Could you check a few things on this model? Use its own coordinates, in mm. Give positions to 0.01 mm unless a question says otherwise; leave off trailing zeros. Order: outer loops, then holes, each group sorted by start corner. A loop starts at its lowest first (then second) coordinate and runs counter-clockwise, first axis right, second up. Notation, with made-up numbers: (-18.75, 23) -> (35.25, 23) arc R29 cw to (35.25, 46) -> close; hole circle Ø4 at (51.25, 69). An arc over 180 degrees is marked (long way). One line per item, written item: value.
```python
from build123d import *

# Parameters (mm, degrees)
CYLINDER_R     = 1.4
CYLINDER_DEPTH = 10
ARRAY001_COUNT = 3
SKETCH018_W    = 3.15
SKETCH018_H    = 2.3
SKETCH002_W    = 5
SKETCH002_H    = 6.8
ARRAY_Z_COUNT  = 6
ARRAY_Z_PITCH  = 1.6
SKETCH005_W    = 10
SKETCH005_H    = 2.2955317108


with BuildPart() as boltholes:
    # Cylinder → Cylinder (new body)
    with BuildSketch(Plane(origin=(0, 6, -1), x_dir=(1, 0, 0), z_dir=(0, 0, 1))):
        Circle(CYLINDER_R)
    extrude(amount=CYLINDER_DEPTH)

    # Array001: BoltHoles ×3 about axis
    array001_axis = Axis((0, 0, 0), (0, 0, 1))


with BuildPart() as boltholes_1:
    add(boltholes.part)
    for i in range(1, ARRAY001_COUNT):
        add(boltholes.part.rotate(array001_axis, i * 360 / ARRAY001_COUNT))


with BuildPart() as obj1:
    # Sketch018 → Revolution007 (revolve)
    with BuildSketch(Plane.XZ):
        with Locations((1.575, 5.7267413876)):
            Rectangle(SKETCH018_W, SKETCH018_H)
    revolve(axis=Axis((0, 0, 0), (0, 0, 1)))


with BuildPart() as obj2:
    # Sketch007 → Revolution006 (revolve)
    with BuildSketch(Plane.XZ):
        with BuildLine():
            ThreePointArc((1.5, 1.7955317108), (0.867020761, 2.4322916436), (0, 2.6655317108))
            Line((0, 2.6655317108), (0, 0.7955317108))
            Line((0, 0.7955317108), (1.5, 0.7955317108))
            Line((1.5, 1.7955317108), (1.5, 0.7955317108))
        make_face()
    revolve(axis=Axis((0, 0, 0), (0, 0, 1)))


with BuildPart() as obj3:
    # Sketch002 → Revolution002 (revolve)
    with BuildSketch(Plane.XZ):
        with Locations((7.5, 3.8)):
            Rectangle(SKETCH002_W, SKETCH002_H)
    revolve(axis=Axis((0, 0, 0), (0, 0, 1)))


with BuildPart() as innergroovetool:
    # Sketch001 → Revolution001 (revolve)
    with BuildSketch(Plane.XZ):
        Polygon((4, 8), (4, 6.4), (8, 6.4), (8.8, 7.2), (8, 8), align=None)
    revolve(axis=Axis((0, 0, 0), (0, 0, 1)))

    # Array Z: InnerGrooveTool ×6


with BuildPart() as innergroovetool_1:
    add(innergroovetool.part)
    with Locations(*[(0, 0, -i * ARRAY_Z_PITCH) for i in range(1, ARRAY_Z_COUNT)]):
        add(innergroovetool.part)

    # Common: intersect obj3
    add(obj3.part, mode=Mode.INTERSECT)


with BuildPart() as clone_of_boltholes001:
    # Sketch → Revolution (revolve)
    with BuildSketch(Plane.XZ):
        Polygon((1.2, 0.4), (8, 0.4), (8, 7.2), (2.8, 7.2), (1.2, 2.2), align=None)
    revolve(axis=Axis((0, 0, 0), (0, 0, 1)))

    # Fusion001: union InnerGrooveTool
    add(innergroovetool_1.part)

    # Cut: cut obj2
    add(obj2.part, mode=Mode.SUBTRACT)

    # Cut003: cut obj1
    add(obj1.part, mode=Mode.SUBTRACT)

    # Cut001: cut BoltHoles
    add(boltholes_1.part, mode=Mode.SUBTRACT)


with BuildPart() as obj4:
    # Sketch005 → Revolution004 (revolve)
    with BuildSketch(Plane.XZ):
        with Locations((5, 0.6477658554)):
            Rectangle(SKETCH005_W, SKETCH005_H)
    revolve(axis=Axis((0, 0, 0), (0, 0, 1)))

    # Common001: intersect Clone of BoltHoles001
    add(clone_of_boltholes001.part, mode=Mode.INTERSECT)


solid = obj4.part
```
1) If I drill on line 1 along Y through (x, z) = (0, 1); line 2 along Y through (x, z) = (0, 0.75); line 3 along X through (y, z) = (-2.25, 0.6), over which ranges is the centre line in solid material (lowest first)?
Answer below:
line 1: y = -8.6 to -1.5, 1.5 to 4.6, 7.4 to 8.6
line 2: y = -8.75 to -1.2, 1.2 to 4.6, 7.4 to 8.75
line 3: x = -8.3 to -6.38, -4.01 to 4.01, 6.38 to 8.3
2) Suppose I cut it at A-A, the plane y = 0. Write out the boundary of the cut face in (x, z).
Answer below:
outline: (-8.8, 0.8) -> (-8.4, 0.4) -> (-1.2, 0.4) -> (-1.2, 0.8) -> (-1.5, 0.8) -> (-1.5, 1.8) -> (-8.2, 1.8) -> (-8, 1.6) -> close; (1.2, 0.4) -> (8.4, 0.4) -> (8.8, 0.8) -> (8, 1.6) -> (8.2, 1.8) -> (1.5, 1.8) -> (1.5, 0.8) -> (1.2, 0.8) -> close
3) Suppose I cut it at B-B, the plane x = 0. Write out the boundary of the cut face in (y, z), then the cut area to 3 significant figures.
Answer below:
outline: (-8.8, 0.8) -> (-8.4, 0.4) -> (-1.2, 0.4) -> (-1.2, 0.8) -> (-1.5, 0.8) -> (-1.5, 1.8) -> (-8.2, 1.8) -> (-8, 1.6) -> close; (1.2, 0.4) -> (4.6, 0.4) -> (4.6, 1.8) -> (1.5, 1.8) -> (1.5, 0.8) -> (1.2, 0.8) -> close; (7.4, 0.4) -> (8.4, 0.4) -> (8.8, 0.8) -> (8, 1.6) -> (8.2, 1.8) -> (7.4, 1.8) -> close
area: 15.6 mm2
4) We'd pull the mould along Y, two halves only. Please class faces 1 (the cylindrical face through (-4.55, -4.24, 1.09)), 2 (the flat face through (-2, 0, 1.796)), 3 (the cylindrical face through (-1.5, 0.07, 1.29)): +Y half, -Y half, draft (parallel to the pull), parting line (faces both ways), or undercut.
Answer below:
face 1: undercut
face 2: draft
face 3: undercut
5) For P1, Ø2, axis at x = 5.2, y = -3, coming from the -Z side; P2, Ø1.5, axis at x = 0.5, y = -0.5, coming from the +Z side, each with a flat end and sliding along its axis, tell me the tip position at first contact or that it passes through.
Answer below:
P1: passes through
P2: stops at z = 0.8
6) Suppose I cut it at C-C, the plane y = -3.5. State how many separate pieces and enclosed holes the cut face has, then the cut area to 3 significant figures.
Answer below:
separate pieces: 3
enclosed holes: 0
area: 14.1 mm2
